Check sheet for the modelled part. Datum: model origin and axes. Units: mm. Face numbers are marked on the shaded views. A direction names the side the tool comes from. Round coordinates to 2 decimals unless told otherwise and drop trailing zeros. Write each loop counter-clockwise with the first axis right and the second up, starting at its lowest first coordinate (ties: lowest second). Pieces come first, ordered by that corner, then holes. Notation, with made-up numbers: M 52,28.5 L 62,28.5 A22 cw 62,56.5 Z; hole C 55,83.5 d4. An arc over 180 degrees is marked long. Answer in a Markdown table with one row per item.
```python
from build123d import *

# Parameters (mm, degrees)
EXTRUDE_307_DEPTH = 17
SKETCH_2_R        = 12.9
EXTRUDE_1_DEPTH   = 60
SKETCH_3_R        = 11
EXTRUDE_2_DEPTH   = 45
FILLET_2_R        = 1
FILLET_4_R        = 0.5


with BuildPart() as part:
    # 草图1 → Extrude 307 (new body)
    with BuildSketch(Plane.XY):
        Polygon((20.984201837, 10.954296262), (1.005402075, 23.65), (-19.978799762, 12.695703738), (-20.984201837, -10.954296262), (-1.005402075, -23.65), (19.978799762, -12.695703738), align=None)
    extrude(amount=EXTRUDE_307_DEPTH)

    # 草图2 → 凸台-拉伸1 (add)
    with BuildSketch(Plane.XY.offset(17)):
        with Locations(Location((0, 0, 0), (0, 0, 180))):
            Circle(SKETCH_2_R)
    extrude(amount=EXTRUDE_1_DEPTH)

    # 草图3 → 凸台-拉伸2 (add)
    with BuildSketch(Plane.XY.offset(77)):
        with Locations(Location((0, 0, 0), (0, 0, 180))):
            Circle(SKETCH_3_R)
    extrude(amount=EXTRUDE_2_DEPTH)

    # 圆角2
    fillet_2_edges = [part.edges().sort_by_distance(p)[0] for p in [
        (11, 0, 122),
    ]]
    fillet(fillet_2_edges, radius=FILLET_2_R)

    # 圆角4
    fillet_4_edges = [part.edges().sort_by_distance(p)[0] for p in [
        (12.9, 0, 77),
    ]]
    fillet(fillet_4_edges, radius=FILLET_4_R)


solid = part.part
```
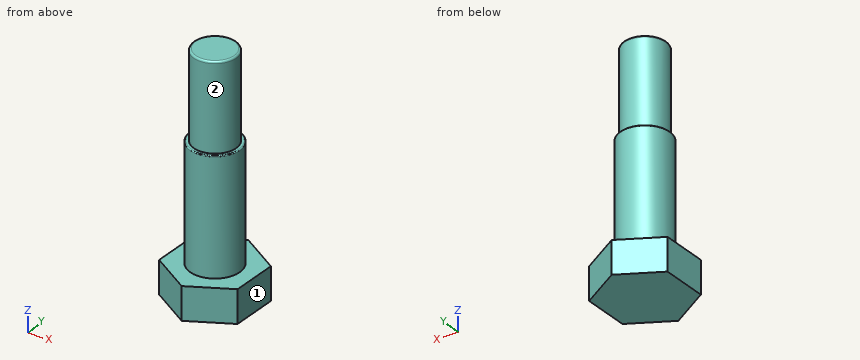
1. Access from +Z, -Z, +X, -X, +Y, -Y to the whole of each face (thin tool, end or side, straight path). Record for the marked faces 1 and 2.
Found:
| item | result |
|---|---|
| face 1 | +Z, -Z, +X, -Y |
| face 2 | +Z |
2. Section check D-D, the plane z = 97. Record the cut outline in (x, y).
Found:
| item | result |
|---|---|
| outline | C 0,0 d22 |
3. Section check C-C, the plane x = 15. Record the cut outline in (y, z), and give its area (3 significant figures).
Found:
| item | result |
|---|---|
| outline | M -15.29,0 L 14.76,0 L 14.76,17 L -15.29,17 Z |
| area | 511 mm2 |
4. Section check B-B, the plane z = 15. Record the cut outline in (x, y), and give its area (3 significant figures).
Found:
| item | result |
|---|---|
| outline | M -20.98,-10.95 L -1.01,-23.65 L 19.98,-12.7 L 20.98,10.95 L 1.01,23.65 L -19.98,12.7 Z |
| area | 1,460 mm2 |
5. Go/stop test with flat-tipped pins: pin 1 (3 mm diameter, centred on x = -5.5, z = 94.5, fed in from +Y); pin 2 (5 mm diameter, centred on x = 5, z = 71, fed in from +Y); pin 3 (1 mm diameter, centred on x = -11.5, y = 8.5, fed in from +Z). Record where each tip stops, or that it passes through.
Found:
| item | result |
|---|---|
| pin 1 | stops at y = 10.25 |
| pin 2 | stops at y = 12.66 |
| pin 3 | stops at z = 17 |
6. Section check A-A, the plane y = 0. Record the cut outline in (x, z), and give its area (3 significant figures).
Found:
| item | result |
|---|---|
| outline | M -20.52,0 L 20.52,0 L 20.52,17 L 12.9,17 L 12.9,76.5 A0.5 ccw 12.4,77 L 11,77 L 11,121 A1 ccw 10,122 L -10,122 A1 ccw -11,121 L -11,77 L -12.4,77 A0.5 ccw -12.9,76.5 L -12.9,17 L -20.52,17 Z |
| area | 3,240 mm2 |
7. Scan lines: L1, parallel to Z at x = -16.5, y = -2; L2, parallel to Y at x = -6.5, z = 68.5; L3, parallel to X at y = -9, z = 19. Record each from-to range of solid material in increasing order.
Found:
| item | result |
|---|---|
| L1 | z = 0 to 17 |
| L2 | y = -11.14 to 11.14 |
| L3 | x = -9.24 to 9.24 |
